The figure shows three views and two pictorial views of one solid part (mm, origin at its lowest corner). Answer the questions. A direction names the side the tool comes from. Give positions to 0.01 mm unless a question says otherwise; leave off trailing zeros. Loops run counter-clockwise (first coordinate to the right, second up) from the corner with the lowest first, then second, coordinate; pieces in that order, holes last. Notation, with made-up numbers: (81.25, -23) -> (90.25, -23) arc R16 cw to (90.25, -17) -> close; hole circle Ø2 at (80.25, 29.25). An arc over 180 degrees is marked (long way). One line per item, written item: value. Start each with the question number.
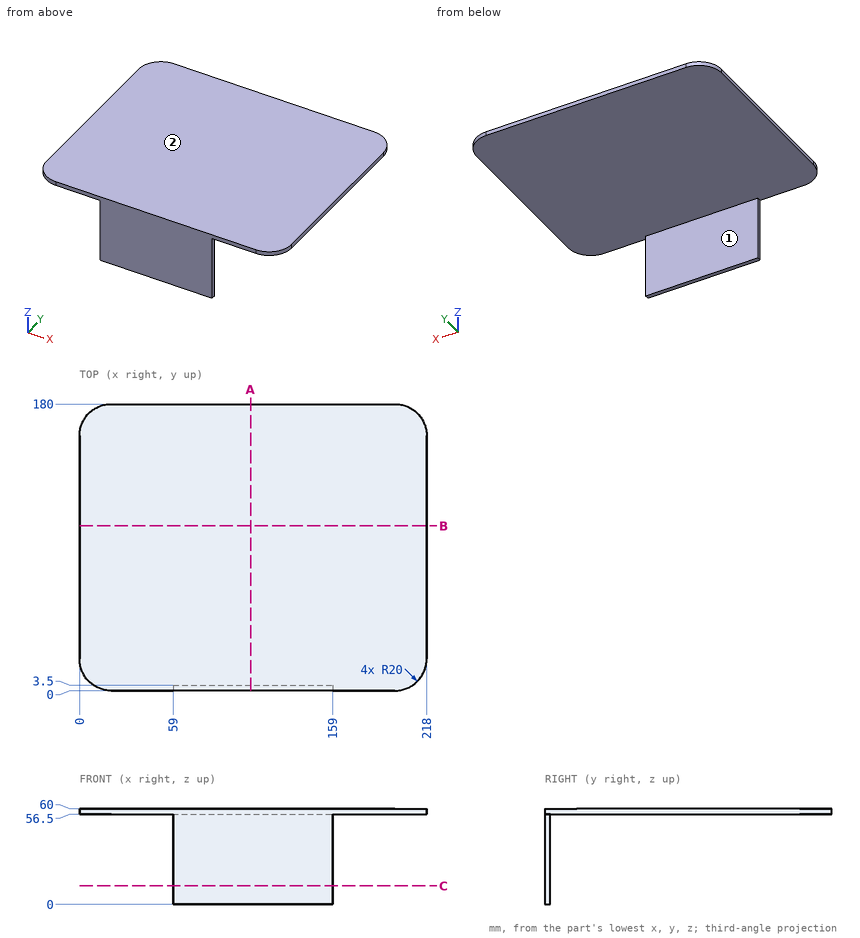
Item 1: Section B-B, the plane y = 103.5 is taken. Determine the outline of the cut face in (x, z), plus the area to 3 significant figures.
Item 2: Section A-A, the plane x = 107.5 is taken. Determine the outline of the cut face in (y, z), plus the area to 3 significant figures.
Item 3: Flat-ended cylindrical pins translate along their axes: pin 1 (4 mm diameter, centred on x = 94.5, y = 62, fed in from -Z); pin 2 (1.8 mm diameter, centred on y = 1, z = 29, fed in from -X); pin 3 (4 mm diameter, centred on y = 2, z = 40, fed in from +X). Find the tip coordinate at first contact, or state that the pin passes through.
Item 4: Consider L1, parallel to Z at x = 145, y = 108; L2, parallel to Y at x = 144, z = 52. Determine where each line is inside the solid, lowest interval first. Write a range as [from, to].
Item 5: Section C-C, the plane z = 11.5 is taken. Determine the outline of the cut face in (x, y), plus the area to 3 significant figures.
Item 6: For the marked faces 1 and 2, determine the directions among +Z, -Z, +X, -X, +Y, -Y from which every point of the face is accessible in a straight line to the end or side of a thin tool.
Computed values:
1. outline: (0, 56.5) -> (218, 56.5) -> (218, 60) -> (0, 60) -> close
1. area: 763 mm²
2. outline: (0, 0) -> (3.5, 0) -> (3.5, 56.5) -> (180, 56.5) -> (180, 60) -> (0, 60) -> close
2. area: 828 mm²
3. pin 1: z = 56.5
3. pin 2: x = 59
3. pin 3: x = 159
4. L1: [56.5, 60]
4. L2: [0, 3.5]
5. outline: (59, 0) -> (159, 0) -> (159, 3.5) -> (59, 3.5) -> close
5. area: 350 mm²
6. face 1: -Z, +X, -X, +Y
6. face 2: +Z, +X, -X, +Y, -Y
